Autodesk Inventor part; units mm, degrees
ref_plane "YZ Plane" through (0, 0, 0) normal (1, 0, 0) x (0, 1, 0)
ref_plane "XZ Plane" through (0, 0, 0) normal (0, 1, 0) x (-1, 0, 0)
ref_plane "XY Plane" through (0, 0, 0) normal (0, 0, 1) x (1, 0, 0)
sketch "Sketch1" plane through (0, 0, 0) normal (0, 1, 0) x (-1, 0, 0)
  line L0 (0, 0) -> (76.2, 0)
  line L1 (0, -76.2) -> (0, 0)
  line L2 (76.2, 0) -> (0, -76.2)
  line L3 (6.35, -6.35) -> (6.35, -58.8833)
  line L4 (58.982, -8.2377) -> (10.1183, -57.1015)
  line L5 (6.35, -6.35) -> (60.8697, -6.35)
  line L6 (60.8697, -6.35) -> (58.982, -8.2377)
  line L7 (6.35, -58.8833) -> (6.35, -60.8697)
  line L8 (6.35, -60.8697) -> (10.1183, -57.1015)
  dimension "d5" = 76.2
  dimension "d6" = 76.2
  dimension "d7" = 6.35
  dimension "d9" = 6.35
extrude "Extrusion1" add sketch "Sketch1" along normal blind 76.2
sketch "Sketch2" plane through (0, 0, 0) normal (1, 0, 0) x (0, 0, -1)
  circle A0 centre (19.05, 19.05) radius 3.3274
  circle A1 centre (57.15, 19.05) radius 3.3274
  circle A2 centre (57.15, 57.15) radius 3.3274
  circle A3 centre (19.05, 57.15) radius 3.3274
  line L0 (0, 76.2) -> (76.2, 76.2)
  line L1 (76.2, 0) -> (76.2, 76.2)
  line L2 (76.2, 0) -> (0, 0)
  line L3 (0, 0) -> (0, 76.2)
  dimension "d12" = 6.6548
  dimension "d13" = 6.6548
  dimension "d14" = 6.6548
  dimension "d15" = 6.6548
  dimension "d16" = 19.05
  dimension "d17" = 19.05
  dimension "d18" = 19.05
  dimension "d19" = 19.05
  dimension "d20" = 19.05
  dimension "d21" = 19.05
  dimension "d22" = 19.05
  dimension "d23" = 19.05
extrude "Extrusion2" cut sketch "Sketch2" against normal blind 25.4 contours A0 | A1 | A2 | A3
sketch "Sketch3" plane through (-76.2, 0, 0) normal (0, 0, 1) x (1, 0, 0)
  circle A0 centre (57.15, 19.05) radius 3.3274
  circle A1 centre (19.05, 19.05) radius 3.3274
  circle A2 centre (19.05, 57.15) radius 3.3274
  circle A3 centre (57.15, 57.15) radius 3.3274
  line L0 (76.2, 0) -> (0, 0)
  line L1 (76.2, 0) -> (76.2, 76.2)
  line L2 (0, 76.2) -> (76.2, 76.2)
  line L3 (0, 0) -> (0, 76.2)
  dimension "d26" = 6.6548
  dimension "d27" = 6.6548
  dimension "d28" = 6.6548
  dimension "d29" = 6.6548
  dimension "d30" = 19.05
  dimension "d31" = 19.05
  dimension "d32" = 19.05
  dimension "d33" = 19.05
  dimension "d34" = 19.05
  dimension "d35" = 19.05
  dimension "d36" = 19.05
  dimension "d37" = 19.05
extrude "Extrusion3" cut sketch "Sketch3" against normal blind 25.4 contours A0 | A1 | A2 | A3
properties part number "15series_3inchCorner"
Can you work these out from the model? Positions are in its coordinate system, mm. A direction names the side the tool comes from. Give positions to 0.01 mm unless a question says otherwise; leave off trailing zeros. Order: outer loops, then holes, each group sorted by start corner. A loop starts at its lowest first (then second) coordinate and runs counter-clockwise, first axis right, second up. Notation, with made-up numbers: M -32,-23 L -23,-23 A11 cw -23,-9 Z; hole C 65.25,86 d7. An arc over 180 degrees is marked long. One line per item, written item: value.
1) I want a section at A-A, the plane y = 23.5. List the corners of the cut face in (x, z) for me.
Answer sheet:
outline: M -76.2,0 L 0,-76.2 L 0,0 Z; hole M -60.87,-6.35 L -58.98,-8.24 L -10.12,-57.1 L -6.35,-60.87 L -6.35,-6.35 Z
2) We'd pull the mould along Z, two halves only. Please class faces 1 (the face through (-60.474, 19.196, -3.131)), 2 (the face through (-3.131, 55.125, -16.409)), 3 (the face through (-38.6, 37.6, -37.6)): released by +Z, released by -Z, zero draft, split by the parting line, or undercut.
Answer sheet:
face 1: zero draft
face 2: undercut
face 3: released by -Z
3) I want a section at B-B, the plane x = -57.15. List the corners of the cut face in (y, z) for me.
Answer sheet:
outline: M 0,-19.05 L 15.72,-19.05 L 15.72,-10.07 L 0,-10.07 Z; M 0,-6.35 L 15.72,-6.35 L 15.72,0 L 0,0 Z; M 22.38,-19.05 L 53.82,-19.05 L 53.82,-10.07 L 22.38,-10.07 Z; M 22.38,-6.35 L 53.82,-6.35 L 53.82,0 L 22.38,0 Z; M 60.48,-19.05 L 76.2,-19.05 L 76.2,-10.07 L 60.48,-10.07 Z; M 60.48,-6.35 L 76.2,-6.35 L 76.2,0 L 60.48,0 Z
4) On a 3-axis mill with a long thin cutter (end or side, diameter ignored), from which of +Z, -Z, +X, -X, +Y, -Y can I reach the whole of each face in a straight line? I mean faces 4 (the face through (-15.976, 17.776, -3.131)), 5 (the face through (-3.131, 17.025, -16.409)), 6 (the face through (-35, 76.2, -35)). Say none if no direction works.
Answer sheet:
face 4: +Z
face 5: +X
face 6: +Z, -Z, +X, -X, +Y
5) Please list where these lines run through material, in increasing order: line 1 along Y through (x, z) = (-57, -2); line 2 along Z through (x, y) = (-2, 19); line 3 along X through (y, z) = (19, -3).
Answer sheet:
line 1: y = 0 to 15.73, 22.37 to 53.83, 60.47 to 76.2
line 2: z = -74.2 to -60.48, -53.82 to -22.38, -15.72 to 0
line 3: x = -73.2 to -60.48, -53.82 to -22.38, -15.72 to 0
6) I want a section at D-D, the plane y = 57.15. Count the separate pieces of the cut face and the enclosed holes in it, plus the area to 3 significant figures.
Answer sheet:
separate pieces: 6
enclosed holes: 0
area: 1,130 mm^2
7) I want a section at C-C, the plane z = -19.05. List the corners of the cut face in (x, y) for me, plus the area to 3 significant figures.
Answer sheet:
outline: M -57.15,0 L -48.17,0 L -48.17,76.2 L -57.15,76.2 L -57.15,60.48 A3.33 cw -57.15,53.82 L -57.15,22.38 A3.33 cw -57.15,15.72 Z; M -6.35,0 L 0,0 L 0,15.72 L -6.35,15.72 Z; M -6.35,22.38 L 0,22.38 L 0,53.82 L -6.35,53.82 Z; M -6.35,60.48 L 0,60.48 L 0,76.2 L -6.35,76.2 Z
area: 1,050 mm^2
8) For P1, Ø6, axis at y = 48.5, z = -26.5, coming from the -X side; P2, Ø5.5, axis at x = -57.15, y = 19.05, coming from the +Z side; P3, Ø10.5, axis at y = 19.05, z = -57.15, coming from the -X side; P4, Ø10.5, axis at y = 57.15, z = -19.05, coming from the -X side, each with a flat end and sliding along its axis, tell me the tip position at first contact or that it passes through.
Answer sheet:
P1: stops at x = -52.7
P2: passes through
P3: stops at x = -24.3
P4: stops at x = -62.4
